The listing builds one solid part. Answer for the finished solid, in the listing's coordinates (mm). Face numbers are marked on the shaded views. A direction names the side the tool comes from. Give positions to 0.01 mm unless a question says otherwise; leave off trailing zeros. Write each loop counter-clockwise with the first axis right and the second up, starting at its lowest first coordinate (ties: lowest second). Pieces come first, ordered by that corner, then holes. Notation, with made-up numbers: (7, -5.75) -> (28, -5.75) arc R10 cw to (28, 13.25) -> close; hole circle Ø6 at (75, 53). An arc over 180 degrees is marked (long way). Put each result on its own line as item: value. Start each with the question number.
1) A cutting plane is placed at D-D (z = 22.5). Write down the section's boundary in (x, y).
2) Flat-ended cylindrical pins translate along their axes: pin 1 Ø2 at (y, z) = (-2, 4) entering from +X; pin 2 Ø0.8 at (y, z) = (1.5, 19) entering from -X; pin 3 Ø2 at (x, y) = (-12, -2) entering from +Z. Find the tip coordinate at first contact, or state that the pin passes through.
3) A cutting plane is placed at B-B (z = 0). Give the number of separate pieces and of enclosed holes in the cut face, then the cut area to 3 significant figures.
4) For the marked faces 1 and 2, determine the directions among +Z, -Z, +X, -X, +Y, -Y from which every point of the face is accessible in a straight line to the end or side of a thin tool.
5) A cutting plane is placed at A-A (x = 0). Write down the section's boundary in (y, z), then the cut area to 3 significant figures.
6) A cutting plane is placed at C-C (y = 2). Write down the section's boundary in (x, z).
7) Find the intervals of material crossed by line 1 along Z through (x, y) = (0, 1.7); line 2 along Y through (x, z) = (9.5, 3); line 3 along X through (y, z) = (1.5, 3), in increasing order. Write a range as from..to.
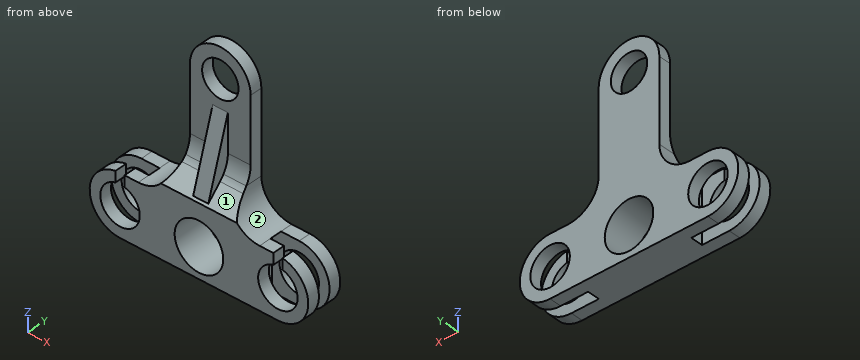
from build123d import *

# Parameters (mm, degrees)
F0_R      = 3.25
F0_R_2    = 4
F0_R_3    = 3
F1_DEPTH  = 3
F2_W      = 9.5
F2_H      = 2
F3_DEPTH  = 10.001
F5_DEPTH  = 2
F6_W      = 4
F6_H      = 5
F7_DEPTH  = 25
F8_DEPTH  = 25
F11_DEPTH = 1.25


with BuildPart() as f1:
    # F0 (on Front) → F1 (new body, symmetric)
    with BuildSketch(Plane.XZ):
        with BuildLine():
            Line((-10, 5), (-13, 5))
            ThreePointArc((-13, 5), (-18, 0), (-13, -5))
            Line((-13, -5), (13, -5))
            ThreePointArc((13, -5), (8, 0), (13, 5))
            Line((13, 5), (10, 5))
            ThreePointArc((10, 5), (6.4644660941, 6.4644660941), (5, 10))
            Line((5, 10), (5, 23.5))
            ThreePointArc((5, 23.5), (0, 28.5), (-5, 23.5))
            Line((-5, 23.5), (-5, 10))
            ThreePointArc((-5, 10), (-6.4644660941, 6.4644660941), (-10, 5))
        make_face()
        with Locations((-13, 0)):
            Circle(F0_R, mode=Mode.SUBTRACT)
        Circle(F0_R_2, mode=Mode.SUBTRACT)
        with Locations((0, 23.5)):
            Circle(F0_R_3, mode=Mode.SUBTRACT)
        with BuildLine():
            ThreePointArc((13, 5), (8, 0), (13, -5))
            ThreePointArc((13, -5), (16.5355339059, -3.5355339059), (18, 0))
            ThreePointArc((18, 0), (16.5355339059, 3.5355339059), (13, 5))
        make_face()
        with Locations((13, 0)):
            Circle(F0_R, mode=Mode.SUBTRACT)
    extrude(amount=F1_DEPTH, both=True)

    # F2 (on face) → F3 (cut, through all)
    with BuildSketch(Plane.XY.offset(5)):
        with Locations((13.25, 0)):
            Rectangle(F2_W, F2_H)
        with Locations((-13.25, 0)):
            Rectangle(F2_W, F2_H)
    extrude(amount=-F3_DEPTH, mode=Mode.SUBTRACT)

    # F4 (on face) → F5 (cut)
    with BuildSketch(Plane.XZ.offset(3)):
        with BuildLine():
            Line((-13.75, 4.9434299833), (-13.75, 3.1622776602))
            ThreePointArc((-13.75, 3.1622776602), (-13, 3.25), (-12.25, 3.1622776602))
            Line((-12.25, 3.1622776602), (-12.25, 5))
            Line((-12.25, 5), (-13, 5))
            ThreePointArc((-13, 5), (-13.3760652094, 4.985837438), (-13.75, 4.9434299833))
        make_face()
        with BuildLine():
            Line((12.25, 5), (12.25, 3.1622776602))
            ThreePointArc((12.25, 3.1622776602), (13, 3.25), (13.75, 3.1622776602))
            Line((13.75, 3.1622776602), (13.75, 4.9434299833))
            ThreePointArc((13.75, 4.9434299833), (13.3760652094, 4.985837438), (13, 5))
            Line((13, 5), (12.25, 5))
        make_face()
    extrude(amount=-F5_DEPTH, mode=Mode.SUBTRACT)

    # F6 (on face) → F7 (cut)
    with BuildSketch(Plane.YZ.offset(5)):
        with BuildLine():
            Line((0.1769726777, 10), (-3, 10))
            Line((-3, 10), (-3, 6.6771860428))
            Line((-3, 6.6771860428), (-0.4644660941, 9.2127199488))
            ThreePointArc((-0.4644660941, 9.2127199488), (-0.1237077096, 9.5900331405), (0.1769726777, 10))
        make_face()
        with BuildLine():
            Line((1, 23.5), (-3, 23.5))
            Line((-3, 23.5), (-3, 10))
            Line((-3, 10), (0.1769726777, 10))
            ThreePointArc((0.1769726777, 10), (0.7898258522, 11.3138312162), (1, 12.7482538547))
            Line((1, 12.7482538547), (1, 23.5))
        make_face()
        with Locations((-1, 26)):
            Rectangle(F6_W, F6_H)
    extrude(amount=-F7_DEPTH, mode=Mode.SUBTRACT)

    # F8 (cut): a face of the model
    f8_faces = [f1.faces().sort_by_distance(p)[0] for p in [
        (5, -1.9067294232, 8.8858021834),
    ]]
    extrude(f8_faces, amount=-F8_DEPTH, mode=Mode.SUBTRACT)

    # F10 (on offset) → F11 (join, symmetric)
    with BuildSketch(Plane.YZ):
        with BuildLine():
            ThreePointArc((0.1769726777, 10), (0.7898258522, 11.3138312162), (1, 12.7482538547))
            Line((1, 12.7482538547), (1, 19))
            Line((1, 19), (-2.6650612591, 7.0121247837))
            Line((-2.6650612591, 7.0121247837), (-0.4644660941, 9.2127199488))
            ThreePointArc((-0.4644660941, 9.2127199488), (-0.1237077096, 9.5900331405), (0.1769726777, 10))
        make_face()
    extrude(amount=F11_DEPTH, both=True)


solid = f1.part
Reply:
1. outline: (-5, 1) -> (-2.83, 1) -> (-2.83, 3) -> (-5, 3) -> close; (2.83, 1) -> (5, 1) -> (5, 3) -> (2.83, 3) -> close
2. pin 1: stops at x = 17
2. pin 2: stops at x = -5
2. pin 3: stops at z = 5
3. separate pieces: 6
3. enclosed holes: 0
3. area: 78.0 mm2
4. face 1: +Z, -Y
4. face 2: +Z, +X, +Y, -Y
5. outline: (-3, -5) -> (3, -5) -> (3, -4) -> (-3, -4) -> close; (-3, 4) -> (3, 4) -> (3, 20.5) -> (1, 20.5) -> (1, 19) -> (-2.67, 7.01) -> (-3, 6.68) -> close; (1, 26.5) -> (3, 26.5) -> (3, 28.5) -> (1, 28.5) -> close
5. area: 77.0 mm2
6. outline: (-13, -5) -> (13, -5) arc R5 ccw to (13, 5) -> (10, 5) arc R5 cw to (5, 10) -> (5, 23.5) arc R5 ccw to (-5, 23.5) -> (-5, 10) arc R5 cw to (-10, 5) -> (-13, 5) arc R5 ccw to start; hole circle Ø6.5 at (-13, 0); hole circle Ø8 at (0, 0); hole circle Ø6 at (0, 23.5); hole circle Ø6.5 at (13, 0)
7. line 1: z = -5..-4, 4..20.5, 26.5..28.5
7. line 2: y = -3..-1, 1..3
7. line 3: x = -17..-14.25, -11.75..-2.65, 2.65..11.75, 14.25..17
